```python
from build123d import *

# Parameters (mm, degrees)
SKETCH1_W           = 352.425
SKETCH1_H           = 152.4
BOSS_EXTRUDE1_DEPTH = 1.5875
CUT_EXTRUDE1_DEPTH  = 4.175
CUT_EXTRUDE2_DEPTH  = 4.175


with BuildPart() as part:
    # Sketch1 → Boss-Extrude1 (new body, symmetric)
    with BuildSketch(Plane(origin=(0, 0, 0), x_dir=(1, 0, 0), z_dir=(0, 1, 0))):
        Rectangle(SKETCH1_W, SKETCH1_H)
    extrude(amount=BOSS_EXTRUDE1_DEPTH, both=True)

    # Sketch2 → Cut-Extrude1 (cut, through all)
    with BuildSketch(Plane(origin=(0, 1.5875, 0), x_dir=(1, 0, 0), z_dir=(0, 1, 0))):
        with BuildLine():
            Line((103.1875, -6.35), (84.1375, -6.35))
            ThreePointArc((84.1375, -6.35), (52.3875, 25.4), (84.1375, 57.15))
            Line((84.1375, 57.15), (103.1875, 57.15))
            ThreePointArc((103.1875, 57.15), (134.9375, 25.4), (103.1875, -6.35))
        make_face()
        with BuildLine():
            Line((-138.1125, 50.8), (-61.9125, 50.8))
            ThreePointArc((-61.9125, 50.8), (-50.179229937, 42.960079591), (-52.932243879, 29.119743879))
            Line((-52.932243879, 29.119743879), (-129.132243879, -47.080256121))
            ThreePointArc((-129.132243879, -47.080256121), (-142.972579591, -49.833270063), (-150.8125, -38.1))
            Line((-150.8125, -38.1), (-150.8125, 38.1))
            ThreePointArc((-150.8125, 38.1), (-147.092756121, 47.080256121), (-138.1125, 50.8))
        make_face()
        with BuildLine():
            Line((-66.270451031, -50.8), (9.929548969, -50.8))
            ThreePointArc((9.929548969, -50.8), (18.90980509, -47.080256121), (22.629548969, -38.1))
            Line((22.629548969, -38.1), (22.629548969, 38.1))
            ThreePointArc((22.629548969, 38.1), (14.78962856, 49.833270063), (0.949292847, 47.080256121))
            Line((0.949292847, 47.080256121), (-75.250707153, -29.119743879))
            ThreePointArc((-75.250707153, -29.119743879), (-78.003721094, -42.960079591), (-66.270451031, -50.8))
        make_face()
    extrude(amount=-CUT_EXTRUDE1_DEPTH, mode=Mode.SUBTRACT)

    # Sketch3 → Cut-Extrude2 (cut, through all)
    with BuildSketch(Plane(origin=(0, 1.5875, 0), x_dir=(1, 0, 0), z_dir=(0, 1, 0))):
        with BuildLine():
            Line((160.3375, -61.9125), (141.2875, -61.9125))
            ThreePointArc((141.2875, -61.9125), (136.525, -57.15), (141.2875, -52.3875))
            Line((141.2875, -52.3875), (160.3375, -52.3875))
            ThreePointArc((160.3375, -52.3875), (165.1, -57.15), (160.3375, -61.9125))
        make_face()
        with BuildLine():
            Line((46.0375, -61.9125), (26.9875, -61.9125))
            ThreePointArc((26.9875, -61.9125), (22.225, -57.15), (26.9875, -52.3875))
            Line((26.9875, -52.3875), (46.0375, -52.3875))
            ThreePointArc((46.0375, -52.3875), (50.8, -57.15), (46.0375, -61.9125))
        make_face()
    extrude(amount=-CUT_EXTRUDE2_DEPTH, mode=Mode.SUBTRACT)


solid = part.part
```
Here's how the part is built. I have some questions about the finished solid (model axes, mm). A direction names the side the tool comes from. Give positions to 0.01 mm unless a question says otherwise; leave off trailing zeros. Order: outer loops, then holes, each group sorted by start corner. A loop starts at its lowest first (then second) coordinate and runs counter-clockwise, first axis right, second up. Notation, with made-up numbers: (38.5, 35) -> (59.5, 35) arc R16 cw to (59.5, 57) -> close; hole circle Ø1 at (8.25, -25). An arc over 180 degrees is marked (long way). Use CSV: the item, a comma, the result in double quotes. Start each with the question number.
Item 1: On a 3-axis mill with a long thin cutter (end or side, diameter ignored), from which of +Z, -Z, +X, -X, +Y, -Y can I reach the whole of each face in a straight line? I mean faces 1 (the flat face through (37, -1.588, -1)), 2 (the flat face through (-36.62, 0.02, -9.51)). Say none if no direction works.
Item 2: Thinking about a two-plate mould opening in X: for faces 3 (the cylindrical face through (14.982, 0.022, -49.752)), 4 (the cylindrical face through (52.395, 0.022, -24.702)), 5 (the flat face through (37, 1.588, -1)), which applies, pulls with the +X half, pulls with the -X half, needs draft (parallel to the pull), parting line crosses it, or undercut?
Item 3: Suppose I cut it at D-D (z = 35). List the corners of the cut face in (x, y) for me.
Item 4: If I drill on probe 1 along X at (y, z) = (-0.05, 58); probe 2 along X at (y, z) = (-1.3, 60); probe 3 along Z at (x, y) = (39, -1.3), over which ranges is the centre line in solid material (lowest first)? Write a range as [from, to].
Item 5: Suppose I cut it at A-A (z = 57.15). List the corners of the cut face in (x, y) for me (1 decimal).
Item 6: Suppose I cut it at C-C (x = -87.5). List the corners of the cut face in (y, z) for me.
Item 7: Suppose I cut it at B-B (z = -6). List the corners of the cut face in (x, y) for me.
Answer block:
1,face 1,"+Z, -Z, +X, -X, -Y"
1,face 2,"+Y, -Y"
2,face 3,"undercut"
2,face 4,"undercut"
2,face 5,"needs draft"
3,outline,"(-176.21, -1.59) -> (-150.81, -1.59) -> (-150.81, 1.59) -> (-176.21, 1.59) -> close; (-117.05, -1.59) -> (-78.59, -1.59) -> (-78.59, 1.59) -> (-117.05, 1.59) -> close; (22.63, -1.59) -> (176.21, -1.59) -> (176.21, 1.59) -> (22.63, 1.59) -> close"
4,probe 1,"x = [-176.21, 22.3], [50.72, 136.6], [165.02, 176.21]"
4,probe 2,"x = [-176.21, 23.17], [49.85, 137.47], [164.15, 176.21]"
4,probe 3,"z = [-76.2, 52.39], [61.91, 76.2]"
5,outline,"(-176.2, -1.6) -> (22.2, -1.6) -> (22.2, 1.6) -> (-176.2, 1.6) -> close; (50.8, -1.6) -> (136.5, -1.6) -> (136.5, 1.6) -> (50.8, 1.6) -> close; (165.1, -1.6) -> (176.2, -1.6) -> (176.2, 1.6) -> (165.1, 1.6) -> close"
6,outline,"(-1.59, -76.2) -> (1.59, -76.2) -> (1.59, -50.8) -> (-1.59, -50.8) -> close; (-1.59, 5.45) -> (1.59, 5.45) -> (1.59, 76.2) -> (-1.59, 76.2) -> close"
7,outline,"(-176.21, -1.59) -> (-150.81, -1.59) -> (-150.81, 1.59) -> (-176.21, 1.59) -> close; (-76.05, -1.59) -> (-40.13, -1.59) -> (-40.13, 1.59) -> (-76.05, 1.59) -> close; (22.63, -1.59) -> (59, -1.59) -> (59, 1.59) -> (22.63, 1.59) -> close; (128.32, -1.59) -> (176.21, -1.59) -> (176.21, 1.59) -> (128.32, 1.59) -> close"
